Geometry check sheet. Reference: the model listing, model coordinates, mm. A direction names the side the tool comes from. Give positions to 0.01 mm unless a question says otherwise; leave off trailing zeros. Write each loop counter-clockwise with the first axis right and the second up, starting at its lowest first coordinate (ties: lowest second). Pieces come first, ordered by that corner, then holes. Notation, with made-up numbers: M 87.25,53 L 130.25,53 A16 cw 130.25,66 Z; hole C 79,-36.75 d10. An arc over 180 degrees is marked long. One line per item, written item: value. Start each with the question number.
1. Gauge pin test, flat ends, axial feed: pin 1 (6 mm diameter, centred on x = -10, y = 15.5, fed in from +Z); pin 2 (2.5 mm diameter, centred on y = 39.5, z = 28, fed in from -X) (3 decimals); pin 3 (4 mm diameter, centred on x = 3.5, z = 23.5, fed in from -Y); pin 4 (3 mm diameter, centred on x = -1.5, z = 35, fed in from +Y). Record the tip position at first contact, or that the pin passes through.
2. Release check for a two-part mould opening along X. For faces 5 (the face through (19, 6, 8)), 6 (the face through (24.11, 8, 4)), 7 (the face through (4, 20, 21)) record: pulls with the +X half, pulls with the -X half, needs draft (parallel to the pull), parting line crosses it, or undercut.
3. Cross-section at B-B on x = 0. Record the cut outline in (y, z) (3 decimals), then the cut area to 3 significant figures.
4. Tool access check on faces 1 (the face through (0, 8.05, 21)), 2 (the face through (-5.5, 19.5, 21.543)), 3 (the face through (0, 39, 36)), 4 (the face through (-0.064, 6.936, 19.581)). Record the directions out of +Z, -Z, +X, -X, +Y, -Y that give a thin tool (end or side, any length) a straight path to the whole face; none if there is none.
5. Scan lines: line 1 (Z direction, x = 5, y = 16.5); line 2 (X direction, y = 40.5, z = 26) (3 decimals); line 3 (Z direction, x = -2.5, y = 21). Record each from-to range of solid material in increasing order.
6. Cross-section at C-C on z = 13.5. Record the cut outline in (x, y).
7. Cross-section at A-A on y = 36. Record the cut outline in (x, z) (3 decimals), then the cut area to 3 significant figures.
8. Cross-section at D-D on x = 20.5. Record the cut outline in (y, z).
from build123d import *

# Parameters (mm, degrees)
SKETCH_1_R                = 17.63
SKETCH_1_R_2              = 14.34
EXTRUDE_1_DEPTH           = 16.05
EXTRUDE_1_2_DEPTH         = 9.77
EXTRUDE_1_2_DEPTH_BACK    = 3
SKETCH_2_W                = 16
SKETCH_2_H                = 16.05
SKETCH_3_W                = 3.41
SKETCH_3_H                = 16
CUT_EXTRUDE_1_DEPTH       = 37.411121927
SKETCH_4_R                = 1.91
CUT_EXTRUDE_2_DEPTH       = 39.675463798
EXTRUDE_2_DEPTH           = 4
EXTRUDE_2_DEPTH_BACK      = 2.77
SKETCH_5_W                = 12.19
SKETCH_5_H                = 8.263625949
SKETCH_6_W                = 12.19
SKETCH_6_H                = 6.77
EXTRUDE_3_DEPTH           = 63
SKETCH_8_W                = 12.19
SKETCH_8_H                = 6.77
EXTRUDE_4_DEPTH           = 0.16
EXTRUDE_5_DEPTH           = 3.16
EXTRUDE_5_DEPTH_BACK      = 10
SKETCH_12_W               = 16
SKETCH_12_H               = 16.05
SKETCH_13_W               = 1.21
SKETCH_13_H               = 16
CUT_EXTRUDE_3_DEPTH       = 73.543164889
SKETCH_14_R               = 1.91
CUT_EXTRUDE_4_DEPTH       = 90.07387176
SKETCH_15_R               = 4.05
CUT_EXTRUDE_5_DEPTH       = 24
SKETCH_16_W               = 56.400519221
SKETCH_16_H               = 19.935010357
CUT_EXTRUDE_6_DEPTH       = 73.088971918
SKETCH_17_W               = 12.19
SKETCH_17_H               = 71.423625949
EXTRUDE_7_DEPTH           = 25
SKETCH_18_W               = 26.793372528
SKETCH_18_H               = 63.398625949
CUT_EXTRUDE_7_DEPTH       = 25
SKETCH_19_R               = 4
CUT_EXTRUDE_8_DEPTH       = 24
CUT_EXTRUDE_9_DEPTH       = 29
EXTRUDE_9_DEPTH           = 2
FILLET_1_R                = 10
SKETCH_24_W               = 12.19
SKETCH_24_H               = 5
EXTRUDE_10_DEPTH          = 27
SKETCH_27_W               = 12.19
SKETCH_27_H               = 10.03
EXTRUDE_11_DEPTH          = 20.23
CUT_EXTRUDE_10_DEPTH      = 45.23
CUT_EXTRUDE_10_DEPTH_BACK = 8
SKETCH_21_W               = 8
SKETCH_21_H               = 16
SKETCH_25_W               = 20.230462415
SKETCH_25_H               = 10.025
CUT_EXTRUDE_12_DEPTH      = 20.23
SKETCH_31_W               = 8
SKETCH_31_H               = 2.03
EXTRUDE_13_DEPTH          = 16.23


with BuildPart() as part:
    # 草圖1 → Extrude 1 (new body)
    with BuildSketch(Plane(origin=(0, 0, 0), x_dir=(1, 0, 0), z_dir=(0, 1, 0))):
        Circle(SKETCH_1_R)
        Circle(SKETCH_1_R_2, mode=Mode.SUBTRACT)
    extrude(amount=EXTRUDE_1_DEPTH)

    # 草圖2 → Extrude 1 2 (add, two sides: drawn at the far end of the back side and taken through both)
    with BuildSketch(Plane(origin=(17.75, 0, 0), x_dir=(0, 0, -1), z_dir=(1, 0, 0)).offset(-EXTRUDE_1_2_DEPTH_BACK)):
        with Locations((0, 8.025)):
            Rectangle(SKETCH_2_W, SKETCH_2_H)
    extrude(amount=EXTRUDE_1_2_DEPTH + EXTRUDE_1_2_DEPTH_BACK)

    # 草圖3 → 除料-伸長1 (cut, through all)
    with BuildSketch(Plane(origin=(0, 16.05, 0), x_dir=(1, 0, 0), z_dir=(0, 1, 0))):
        with Locations((25.815, 0)):
            Rectangle(SKETCH_3_W, SKETCH_3_H)
    extrude(amount=-CUT_EXTRUDE_1_DEPTH, mode=Mode.SUBTRACT)

    # 草圖4 → 除料-伸長2 (cut, through all)
    with BuildSketch(Plane.XY.offset(8)):
        with Locations((19.910203689, 8.025)):
            Circle(SKETCH_4_R)
    extrude(amount=-CUT_EXTRUDE_2_DEPTH, mode=Mode.SUBTRACT)

    # 草圖5 → 填料-伸長2 (add, two sides: drawn at the far end of the back side and taken through both)
    with BuildSketch(Plane.XY.offset(17.75).offset(-EXTRUDE_2_DEPTH_BACK)):
        with Locations((0, 12.156812974)):
            Rectangle(SKETCH_5_W, SKETCH_5_H)
    extrude(amount=EXTRUDE_2_DEPTH + EXTRUDE_2_DEPTH_BACK)

    # 草圖6 → 填料-伸長3 (add)
    with BuildSketch(Plane(origin=(0, 16.288625949, 0), x_dir=(1, 0, 0), z_dir=(0, 1, 0))):
        with Locations((0, -18.365)):
            Rectangle(SKETCH_6_W, SKETCH_6_H)
    extrude(amount=EXTRUDE_3_DEPTH)

    # 草圖8 → 填料-伸長4 (add)
    with BuildSketch(Plane(origin=(0, 79.288625949, 0), x_dir=(1, 0, 0), z_dir=(0, 1, 0))):
        with Locations((0, -18.365)):
            Rectangle(SKETCH_8_W, SKETCH_8_H)
    extrude(amount=EXTRUDE_4_DEPTH)

    # 草圖12 → 填料-伸長5 (add, two sides: drawn at the far end of the back side and taken through both)
    with BuildSketch(Plane(origin=(-17.75, 0, 0), x_dir=(0, 0, -1), z_dir=(1, 0, 0)).offset(-EXTRUDE_5_DEPTH_BACK)):
        with Locations((0.543544944, 8.025)):
            Rectangle(SKETCH_12_W, SKETCH_12_H)
    extrude(amount=EXTRUDE_5_DEPTH + EXTRUDE_5_DEPTH_BACK)

    # 草圖13 → 除料-伸長3 (cut, through all)
    with BuildSketch(Plane(origin=(0, 16.05, 0), x_dir=(1, 0, 0), z_dir=(0, 1, 0))):
        with Locations((-27.145, 0.543544944)):
            Rectangle(SKETCH_13_W, SKETCH_13_H)
    extrude(amount=-CUT_EXTRUDE_3_DEPTH, mode=Mode.SUBTRACT)

    # 草圖14 → 除料-伸長4 (cut, through all)
    with BuildSketch(Plane(origin=(0, 0, -8.543544944), x_dir=(-1, 0, 0), z_dir=(0, 0, -1))):
        with Locations(Location((20.980783679, 8.025, 0), (0, 0, 90))):
            Circle(SKETCH_14_R)
    extrude(amount=-CUT_EXTRUDE_4_DEPTH, mode=Mode.SUBTRACT)

    # 草圖15 → 除料-伸長5 (cut)
    with BuildSketch(Plane(origin=(0, 79.448625949, 0), x_dir=(1, 0, 0), z_dir=(0, 1, 0))):
        with Locations((0, -14.98)):
            Circle(SKETCH_15_R)
    extrude(amount=-CUT_EXTRUDE_5_DEPTH, mode=Mode.SUBTRACT)

    # 草圖16 → 除料-伸長6 (cut, through all)
    with BuildSketch(Plane(origin=(0, 16.05, 0), x_dir=(1, 0, 0), z_dir=(0, 1, 0))):
        with Locations((-4.090259611, 9.967505179)):
            Rectangle(SKETCH_16_W, SKETCH_16_H)
    extrude(amount=-CUT_EXTRUDE_6_DEPTH, mode=Mode.SUBTRACT)

    # 草圖17 → 填料-伸長7 (add)
    with BuildSketch(Plane.XY.offset(21.75)):
        with Locations((0, 43.736812975)):
            Rectangle(SKETCH_17_W, SKETCH_17_H)
    extrude(amount=EXTRUDE_7_DEPTH)

    # 草圖18 → 除料-伸長7 (cut)
    with BuildSketch(Plane.ZY.offset(6.095)):
        with Locations((28.376686264, 47.749312975)):
            Rectangle(SKETCH_18_W, SKETCH_18_H)
    extrude(amount=-CUT_EXTRUDE_7_DEPTH, mode=Mode.SUBTRACT)

    # 草圖19 → 除料-伸長8 (cut)
    with BuildSketch(Plane(origin=(0, 79.448625949, 0), x_dir=(1, 0, 0), z_dir=(0, 1, 0))):
        with Locations((0, -41.773372528)):
            Circle(SKETCH_19_R)
    extrude(amount=-CUT_EXTRUDE_8_DEPTH, mode=Mode.SUBTRACT)

    # 草圖20 → 除料-伸長9 (cut)
    with BuildSketch(Plane(origin=(6.095, 0, 0), x_dir=(0, 0, -1), z_dir=(1, 0, 0))):
        Polygon((-41.773372528, 16.05), (-41.773372528, 8.025), (-46.75, 8.025), (-46.75, 79.448625949), (-41.773372528, 79.448625949), align=None)
    extrude(amount=-CUT_EXTRUDE_9_DEPTH, mode=Mode.SUBTRACT)

    # 草圖23 → 填料-伸長9 (add)
    with BuildSketch(Plane.XZ.offset(-8.025)):
        Polygon((-6.095, 41.773372528), (-6.095, 17.75), (6.13829314, 17.75), (6.095, 41.773372528), align=None)
    extrude(amount=EXTRUDE_9_DEPTH)

    # 圓角1
    # the kernel refuses this fillet: 10 mm, written as the material it takes off along each edge
    with BuildSketch(Plane(origin=(-21.095, 6.025, 17.75), x_dir=(0, 1, 0), z_dir=(1, 0, 0))) as fillet_1_piece_1:
        with BuildLine():
            CenterArc((10, 6), FILLET_1_R, 180, 36.869897646)
            Line((0, 6), (0, 0))
            Line((0, 0), (2, 0))
        make_face()
    extrude(amount=42.23329314, mode=Mode.SUBTRACT)

    # 草圖24 → 填料-伸長10 (add)
    with BuildSketch(Plane(origin=(0, 16.05, 0), x_dir=(1, 0, 0), z_dir=(0, 1, 0))):
        with Locations((0, -19.042910113)):
            Rectangle(SKETCH_24_W, SKETCH_24_H)
    extrude(amount=EXTRUDE_10_DEPTH)

    # 草圖27 → 填料-伸長11 (add)
    with BuildSketch(Plane.XY.offset(21.542910113)):
        with Locations((0, 38.035)):
            Rectangle(SKETCH_27_W, SKETCH_27_H)
    extrude(amount=EXTRUDE_11_DEPTH)

    # 草圖21 → 除料-伸長10 (cut, two sides: drawn at the far end of the back side and taken through both)
    with BuildSketch(Plane(origin=(0, 16.05, 0), x_dir=(1, 0, 0), z_dir=(0, 1, 0)).offset(-CUT_EXTRUDE_10_DEPTH_BACK)):
        with Locations((0, -28)):
            Rectangle(SKETCH_21_W, SKETCH_21_H)
    extrude(amount=CUT_EXTRUDE_10_DEPTH + CUT_EXTRUDE_10_DEPTH_BACK, mode=Mode.SUBTRACT)

    # 草圖25 → 除料-伸長12 (cut)
    with BuildSketch(Plane.ZY.offset(6.095)):
        with Locations((31.658141321, 11.0375)):
            Rectangle(SKETCH_25_W, SKETCH_25_H)
    extrude(amount=-CUT_EXTRUDE_12_DEPTH, mode=Mode.SUBTRACT)

    # 草圖31 → 填料-伸長13 (add)
    with BuildSketch(Plane(origin=(0, 0, 36), x_dir=(-1, 0, 0), z_dir=(0, 0, -1))):
        with Locations((0, 34.035)):
            Rectangle(SKETCH_31_W, SKETCH_31_H)
    extrude(amount=EXTRUDE_13_DEPTH)


solid = part.part
Report:
1. pin 1: stops at z = 16.18
1. pin 2: stops at x = -6.095
1. pin 3: stops at y = 6.27
1. pin 4: stops at y = 43.05
2. face 5: needs draft
2. face 6: pulls with the +X half
2. face 7: undercut
3. outline: M 0,14.34 L 16.05,14.34 L 16.05,16.543 L 43.05,16.543 L 43.05,20 L 35.05,20 L 35.05,36 L 43.05,36 L 43.05,41.773 L 33.02,41.773 L 33.02,20 L 8.05,20 L 8.05,21.543 L 6.272,21.543 A10 ccw 8.025,17.75 L 8.025,17.63 L 0,17.63 Z
3. area: 260 mm^2
4. face 1: +Z
4. face 2: +Z, +X, -X, -Y
4. face 3: +Y
4. face 4: +X, -X, -Y
5. line 1: z = 16.54 to 21.54
5. line 2: x = -6.095 to -4, 4 to 6.095
5. line 3: z = 16.54 to 20
6. outline: M -11.34,0 L -4.84,0 L -4.84,16.05 L -11.34,16.05 Z; M 4.84,0 L 11.34,0 L 11.34,16.05 L 4.84,16.05 Z
7. outline: M -6.095,16.543 L 6.095,16.543 L 6.095,41.773 L -6.095,41.773 Z; hole M -4,20 L 4,20 L 4,36 L -4,36 Z
7. area: 180 mm^2
8. outline: M 0,0 L 6.21,0 L 6.21,8 L 0,8 Z; M 9.84,0 L 16.05,0 L 16.05,8 L 9.84,8 Z
